The model under review builds one solid part; all positions refer to its coordinate system, in mm. Give positions to 0.01 mm unless a question says otherwise; leave off trailing zeros. Order: outer loops, then holes, each group sorted by start corner. A loop starts at its lowest first (then second) coordinate and runs counter-clockwise, first axis right, second up. Notation, with made-up numbers: (74.5, -1.5) - (91.5, -1.5) arc R19 cw to (91.5, 30.5) - close; hole circle Ø10 at (82, 56). An arc over 180 degrees is marked (long way). Write item = value, one per line. Start each with the question number.
1. We need section B-B, the plane x = -23.5. Give the boundary of the cut face in (y, z), and give its area (3 significant figures).
2. For P1, Ø10, axis at x = -4.5, z = 49, coming from the -Y side, flat-tipped, find the tip position at first contact; note if it passes through.
3. We need section A-A, the plane z = 14. Give the boundary of the cut face in (x, y), and give its area (3 significant figures).
4. Wall thickness on probe 1 along Z at (x, y) = (-23.5, 0.75); probe 2 along X at (y, z) = (0.9, 88); probe 3 along X at (y, z) = (1.3, 12.5): over which ranges is each line inside the solid? List them lowest first.
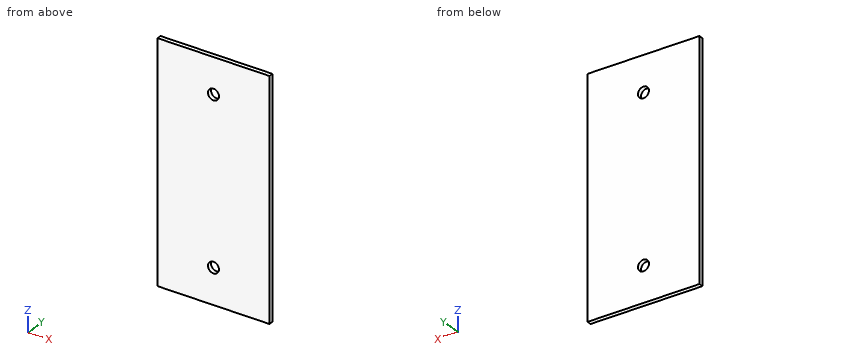
Autodesk Inventor part; units mm, degrees
ref_plane "YZ Plane" through (0, 0, 0) normal (1, 0, 0) x (0, 1, 0)
ref_plane "XZ Plane" through (0, 0, 0) normal (0, 1, 0) x (-1, 0, 0)
ref_plane "XY Plane" through (0, 0, 0) normal (0, 0, 1) x (1, 0, 0)
sketch "Sketch1" plane through (0, 0, 0) normal (0, 1, 0) x (-1, 0, 0)
  line L0 (0, 0) -> (47, 0)
  line L1 (47, 0) -> (47, 102)
  line L2 (47, 102) -> (0, 102)
  line L3 (0, 102) -> (0, 0)
  line L4 (47, 0) -> (49, 0)
  line L5 (49, 0) -> (49, -2)
  line L6 (49, -2) -> (47, -2)
  line L7 (47, -2) -> (47, 0)
  line L8 (47, 102) -> (49, 102)
  line L9 (49, 102) -> (49, 104)
  line L10 (49, 104) -> (47, 104)
  line L11 (47, 104) -> (47, 102)
  line L12 (0, 102) -> (-2, 102)
  line L13 (-2, 102) -> (-2, 104)
  line L14 (-2, 104) -> (0, 104)
  line L15 (0, 104) -> (0, 102)
  line L16 (0, 0) -> (-2, 0)
  line L17 (-2, 0) -> (-2, -2)
  line L18 (-2, -2) -> (0, -2)
  line L19 (0, -2) -> (0, 0)
  line L20 (47, -2) -> (0, -2)
  line L21 (-2, 0) -> (-2, 102)
  line L22 (0, 104) -> (47, 104)
  line L23 (49, 102) -> (49, 0)
  line L24 (23.5, 102) -> (23.5, 90.5)
  line L25 (23.5, 90.5) -> (23.5, 88)
  circle A0 centre (23.5, 88) radius 2.5
  line L26 (47, 51) -> (0, 51)
  circle A1 centre (23.5, 14) radius 2.5
  dimension "d14" = 47
  dimension "d15" = 102
  dimension "d16" = 2
  dimension "d17" = 2
  dimension "d18" = 2
  dimension "d19" = 2
  dimension "d20" = 2
  dimension "d21" = 2
  dimension "d22" = 2
  dimension "d23" = 2
  dimension "d28" = 11.5
  dimension "d29" = 2.5
sketch "Sketch2" plane through (0, 0, 0) normal (1, 0, 0) x (0, 1, 0)
  point P0 (0, 0)
extrude "Extrusion1" add sketch "Sketch1" along normal blind 2
sketch "Sketch3" plane through (2, 0, 104) normal (1, 0, 0) x (0, 0, -1)
  point P0 (104, 0)
sketch "Sketch4" plane through (2, 0, 104) normal (1, 0, 0) x (0, 0, -1)
  line L0 (106, 0) -> (0, 0)
  line L1 (0, 0) -> (2, 0)
  line L2 (2, 0) -> (2, 2)
  line L3 (2, 2) -> (0, 2)
  line L4 (0, 2) -> (0, 0)
  line L5 (2, 0) -> (104, 0)
  line L6 (104, 0) -> (104, -40)
  line L7 (104, -40) -> (2, -40)
  line L8 (2, -40) -> (2, 0)
  line L9 (2, -40) -> (0, -40)
  line L10 (0, -40) -> (0, -42)
  line L11 (0, -42) -> (2, -42)
  line L12 (2, -42) -> (2, -40)
  line L13 (104, -40) -> (106, -40)
  line L14 (106, -40) -> (106, -42)
  line L15 (106, -42) -> (104, -42)
  line L16 (104, -42) -> (104, -40)
  line L17 (104, 0) -> (106, 0)
  line L18 (106, 0) -> (106, 2)
  line L19 (106, 2) -> (104, 2)
  line L20 (104, 2) -> (104, 0)
  line L21 (0, 0) -> (0, -40)
  line L22 (2, -42) -> (104, -42)
  line L23 (106, -40) -> (106, 0)
  line L24 (2, 2) -> (104, 2)
  dimension "d33" = 2
  dimension "d34" = 2
  dimension "d35" = 102
  dimension "d36" = 40
  dimension "d37" = 2
  dimension "d38" = 2
  dimension "d39" = 2
  dimension "d40" = 2
  dimension "d41" = 2
  dimension "d42" = 2
sketch "Sketch5" plane through (0, 0, 0) normal (0, 0, 1) x (1, 0, 0)
  point P0 (0, 0)
equation "\"d14\" = largeur_ins"
equation "\"d15\" = longueur_ins"
equation "\"d16\" = epaisseur"
equation "\"d17\" = epaisseur"
equation "\"d18\" = epaisseur"
equation "\"d19\" = epaisseur"
equation "\"d20\" = epaisseur"
equation "\"d21\" = epaisseur"
equation "\"d22\" = epaisseur"
equation "\"d23\" = epaisseur"
equation "\"d31\" = epaisseur"
equation "\"d33\" = epaisseur"
equation "\"d34\" = epaisseur"
equation "\"d35\" = longueur_ins"
equation "\"d36\" = hauteur_inside"
equation "\"d37\" = epaisseur"
equation "\"d38\" = epaisseur"
equation "\"d39\" = epaisseur"
equation "\"d40\" = epaisseur"
equation "\"d41\" = epaisseur"
equation "\"d42\" = epaisseur"
equation "\"epaisseur\" = 2"
equation "\"largeur_ins\" = 47"
equation "\"longueur_ins\" = 102"
equation "\"dist_laser\" = 69"
equation "\"hauteur_inside\" = 40"
properties part number "boitier_laser"
Model answer:
q1.outline = (0, -2) - (2, -2) - (2, 11.5) - (0, 11.5) - close; (0, 16.5) - (2, 16.5) - (2, 85.5) - (0, 85.5) - close; (0, 90.5) - (2, 90.5) - (2, 104) - (0, 104) - close
q1.area = 192 mm2
q2.P1 = 0
q3.outline = (-49, 0) - (-26, 0) - (-26, 2) - (-49, 2) - close; (-21, 0) - (2, 0) - (2, 2) - (-21, 2) - close
q3.area = 92.0 mm2
q4.probe_1 = -2 to 11.5, 16.5 to 85.5, 90.5 to 104
q4.probe_2 = -49 to -26, -21 to 2
q4.probe_3 = -49 to -25.5, -21.5 to 2
